Can you work these out from the model? Positions are in its coordinate system, mm. Face numbers are marked on the shaded views. A direction names the side the tool comes from. Round coordinates to 2 decimals unless told otherwise and drop trailing zeros. Loops run counter-clockwise (first coordinate to the right, second up) from the corner with the lowest first, then second, coordinate; pieces in that order, holes last. Notation, with made-up numbers: (12.5, 67.25) -> (54.5, 67.25) arc R28 cw to (54.5, 100.25) -> close; hole circle Ø9 at (25, -33.5). An arc over 180 degrees is marked (long way). Write each question's results on one line, items separated by ' | '.
from build123d import *

# Parameters (mm, degrees)
F1_DEPTH = 6.3625
F2_R     = 2
F2_R_2   = 1.6
F3_DEPTH = 14.288708


with BuildPart() as f1:
    # F0 (on Right) → F1 (new body, symmetric)
    with BuildSketch(Plane.YZ):
        with BuildLine():
            Line((40, -6.35), (40, 6.35))
            Line((40, 6.35), (12.5, 6.35))
            ThreePointArc((12.5, 6.35), (0, 7.937708), (-12.5, 6.35))
            Line((-12.5, 6.35), (-40, 6.35))
            Line((-40, 6.35), (-40, -6.35))
            Line((-40, -6.35), (-12.5, -6.35))
            ThreePointArc((-12.5, -6.35), (0, -7.937708), (12.5, -6.35))
            Line((12.5, -6.35), (40, -6.35))
        make_face()
        with BuildLine():
            ThreePointArc((1.601021, 2.5), (12, 0), (1.601021, -2.5))
            Line((1.601021, -2.5), (-1.601021, -2.5))
            ThreePointArc((-1.601021, -2.5), (-12, 0), (-1.601021, 2.5))
            Line((-1.601021, 2.5), (1.601021, 2.5))
        make_face(mode=Mode.SUBTRACT)
    extrude(amount=F1_DEPTH, both=True)

    # F2 (on face) → F3 (cut, through all)
    with BuildSketch(Plane.XY.offset(6.35)):
        with Locations((0, -20)):
            Circle(F2_R)
        with Locations((0, -35)):
            Circle(F2_R)
        with Locations((0, 20)):
            Circle(F2_R_2)
        with Locations((0, 35)):
            Circle(F2_R_2)
        Polygon((6.3625, 27.25), (6.3625, 27.75), (5.929487, 27.5), align=None)
        Polygon((-5.929487, 27.5), (-6.3625, 27.75), (-6.3625, 27.25), align=None)
    extrude(amount=-F3_DEPTH, mode=Mode.SUBTRACT)


solid = f1.part
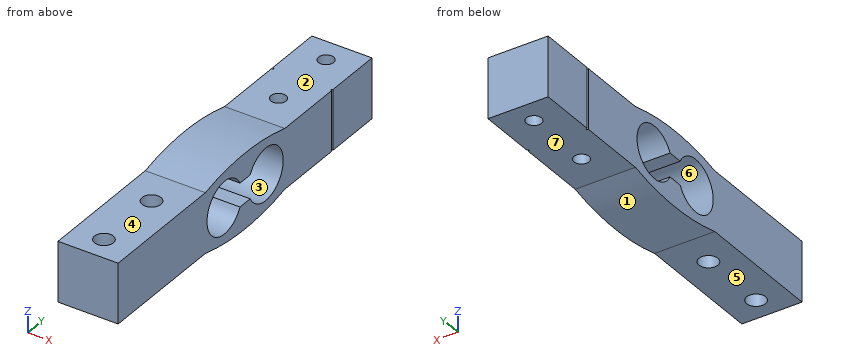
1. If we section it at A-A (z = 0): List the corners of the cut face in (x, y) for me.
Final values:
outline: (-6.36, -40) -> (6.36, -40) -> (6.36, -12) -> (-6.36, -12) -> close; (-6.36, 12) -> (6.36, 12) -> (6.36, 27.25) -> (5.93, 27.5) -> (6.36, 27.75) -> (6.36, 40) -> (-6.36, 40) -> (-6.36, 27.75) -> (-5.93, 27.5) -> (-6.36, 27.25) -> close; hole circle Ø4 at (0, -35); hole circle Ø4 at (0, -20); hole circle Ø3.2 at (0, 20); hole circle Ø3.2 at (0, 35)
2. On a 3-axis mill with a long thin cutter (end or side, diameter ignored), from which of +Z, -Z, +X, -X, +Y, -Y can I reach the whole of each face in a straight line? I mean the marked faces 4, 5, 6 and 7. Say none if no direction works.
Final values:
face 4: +Z, +X, -X, -Y | face 5: -Z, +X, -X, -Y | face 6: +X, -X | face 7: -Z, +X, -X, +Y
3. If we section it at D-D (z = 3.25): List the corners of the cut face in (x, y) for me.
Final values:
outline: (-6.36, -40) -> (6.36, -40) -> (6.36, -10.94) -> (-6.36, -10.94) -> close; (-6.36, -2.06) -> (6.36, -2.06) -> (6.36, 2.06) -> (-6.36, 2.06) -> close; (-6.36, 10.94) -> (6.36, 10.94) -> (6.36, 27.25) -> (5.93, 27.5) -> (6.36, 27.75) -> (6.36, 40) -> (-6.36, 40) -> (-6.36, 27.75) -> (-5.93, 27.5) -> (-6.36, 27.25) -> close; hole circle Ø4 at (0, -35); hole circle Ø4 at (0, -20); hole circle Ø3.2 at (0, 20); hole circle Ø3.2 at (0, 35)
4. We'd pull the mould along Z, two halves only. Please class the marked faces 1, 2 and 3: pulls with the +Z half, pulls with the -Z half, needs draft (parallel to the pull), parting line crosses it, or undercut.
Final values:
face 1: pulls with the -Z half | face 2: pulls with the +Z half | face 3: undercut
5. If we section it at B-B (y = 20): List the corners of the cut face in (x, z) for me, then the cut area to 3 significant figures.
Final values:
outline: (-6.36, -6.35) -> (-1.6, -6.35) -> (-1.6, 6.35) -> (-6.36, 6.35) -> close; (1.6, -6.35) -> (6.36, -6.35) -> (6.36, 6.35) -> (1.6, 6.35) -> close | area: 121 mm2
6. Will these pins go through, and if not, where does the flat tip stop? pin 1 (4.5 mm diameter, centred on x = 0, y = -35, fed in from +Z); pin 2 (4 mm diameter, centred on x = -4, y = -14, fed in from +Z); pin 3 (5 mm diameter, centred on x = 0, y = 20, fed in from -Z).
Final values:
pin 1: z = 6.35 | pin 2: z = 6.48 | pin 3: z = -6.35
7. If we section it at C-C (x = 5.25): List the corners of the cut face in (y, z) for me.
Final values:
outline: (-40, -6.35) -> (-12.5, -6.35) arc R50 ccw to (12.5, -6.35) -> (40, -6.35) -> (40, 6.35) -> (12.5, 6.35) arc R50 ccw to (-12.5, 6.35) -> (-40, 6.35) -> close; hole (-1.6, -2.5) -> (1.6, -2.5) arc R5.5 ccw (long way) to (1.6, 2.5) -> (-1.6, 2.5) arc R5.5 ccw (long way) to start
8. Please list where these lines run through material, in increasing order: line 1 (Y direction, x = -0.25, z = 1.25); line 2 (Y direction, x = 4.25, z = -3.75); line 3 (Z direction, x = -5.5, y = 1). Write a range as from..to.
Final values:
line 1: -40..-36.98, -33.02..-21.98, -18.02..-11.86, 11.86..18.42, 21.58..33.42, 36.58..40 | line 2: -40..-10.52, -2.48..2.48, 10.52..40 | line 3: -7.93..-2.5, 2.5..7.93
